The drawing under review shows one solid part. Ordinate dimensions are in mm from its lowest x, y, z. A direction names the side the tool comes from. Round coordinates to 2 decimals unless told otherwise and drop trailing zeros. Loops run counter-clockwise (first coordinate to the right, second up) from the corner with the lowest first, then second, coordinate; pieces in that order, holes last. Notation, with made-up numbers: M -13,-2 L 8,-2 A8 ccw 8,6 Z; hole C -22.75,43 d5. An arc over 180 degrees is marked long. Use a Markdown table: item, result.
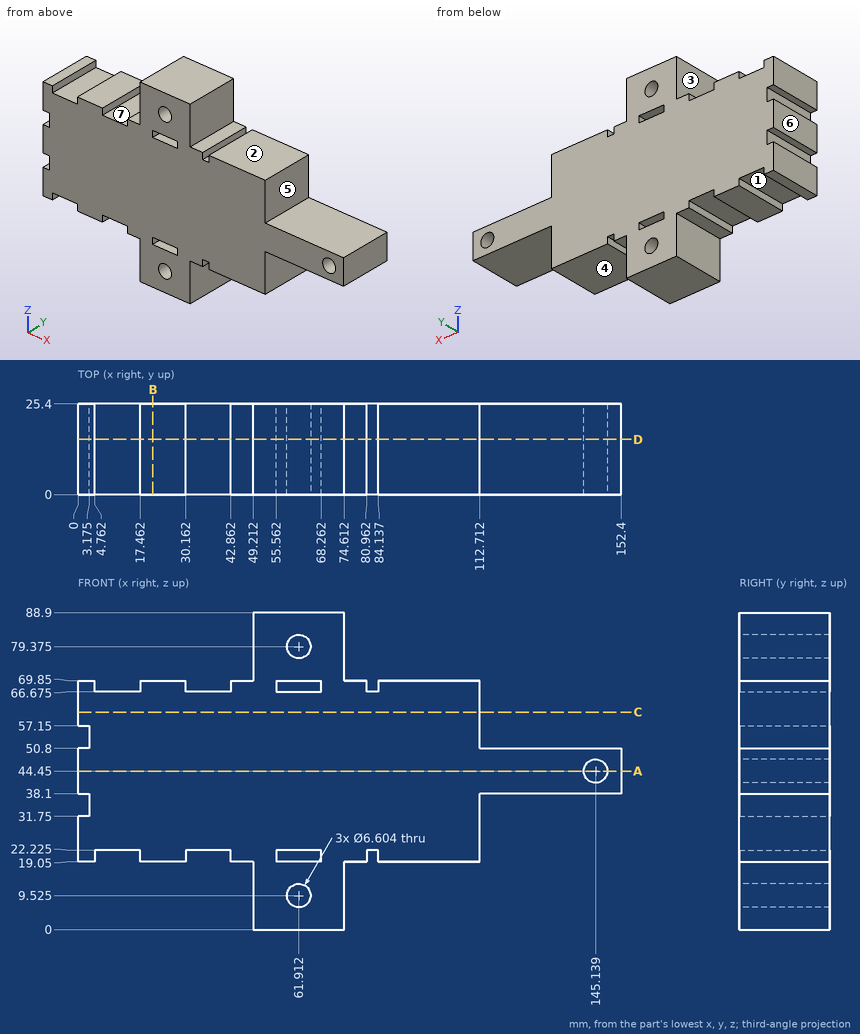
1. Take a section at B-B on x = 21. Give the boundary of the cut face in (y, z), and give its area (3 significant figures).
Check values:
| item | result |
|---|---|
| outline | M 0,19.05 L 25.4,19.05 L 25.4,69.85 L 0,69.85 Z |
| area | 1,290 mm² |
2. The part is to be moulded in two halves that separate along X. For the marked faces 5, 6 and 7, say which applies: pulls with the +X half, pulls with the -X half, needs draft (parallel to the pull), parting line crosses it, or undercut.
Check values:
| item | result |
|---|---|
| face 5 | pulls with the +X half |
| face 6 | pulls with the -X half |
| face 7 | undercut |
3. Take a section at C-C on z = 61. Give the boundary of the cut face in (x, y).
Check values:
| item | result |
|---|---|
| outline | M 0,0 L 112.71,0 L 112.71,25.4 L 0,25.4 Z |
4. Take a section at A-A on z = 44.45. Give the boundary of the cut face in (x, y).
Check values:
| item | result |
|---|---|
| outline | M 0,0 L 141.84,0 L 141.84,25.4 L 0,25.4 Z; M 148.44,0 L 152.4,0 L 152.4,25.4 L 148.44,25.4 Z |
5. Wall thickness on line 1 along X through (y, z) = (17.75, 69); line 2 along X through (y, z) = (8.5, 54) (1 decimal); line 3 along Z through (x, y) = (138.5, 21): over which ranges is each line inside the solid? List them lowest first. Write a range as from..to.
Check values:
| item | result |
|---|---|
| line 1 | x = 0..4.76, 17.46..30.16, 42.86..55.56, 68.26..80.96, 84.14..112.71 |
| line 2 | x = 3.2..112.7 |
| line 3 | z = 38.1..50.8 |
6. Take a section at D-D on y = 15.5. Count the separate pieces of the cut face and the enclosed holes in it, and give its area (3 significant figures).
Check values:
| item | result |
|---|---|
| separate pieces | 1 |
| enclosed holes | 5 |
| area | 6,790 mm² |
7. Machinability: for the marked faces 1, 2, 3 and 4, which of the approach directions +Z, -Z, +X, -X, +Y, -Y give a long, thin tool a straight path to every point of the face, cutting with its end or side? Answer none if there is none.
Check values:
| item | result |
|---|---|
| face 1 | -Z, +Y, -Y |
| face 2 | +Z, +X, +Y, -Y |
| face 3 | +Z, -X, +Y, -Y |
| face 4 | -Z, +X, +Y, -Y |
8. Insertion check: pin 1 (10 mm diameter, centred on y = 16, z = 9, fed in from -X); pin 2 (3.5 mm diameter, centred on y = 16.5, z = 69, fed in from +X); pin 3 (6.5 mm diameter, centred on x = 35.5, y = 9.5, fed in from +Z) (1 decimal). Each pin has a flat end and moves straight along its axis. Give the tip position at first contact, or say it passes through.
Check values:
| item | result |
|---|---|
| pin 1 | stops at x = 49.21 |
| pin 2 | stops at x = 112.71 |
| pin 3 | stops at z = 66.7 |
